from build123d import *

# Parameters (mm, degrees)
SKETCH_1_W           = 14
SKETCH_1_H           = 22
EXTRUDE_1_DEPTH      = 5
SKETCH_2_OUTSIDE_W   = 21.31
SKETCH_2_OUTSIDE_H   = 29.31
SKETCH_2_OUTSIDE_W_2 = 11
SKETCH_2_OUTSIDE_H_2 = 19
CUT_EXTRUDE_1_DEPTH  = 3.5
SKETCH_3_W           = 8
SKETCH_3_H           = 16
CUT_EXTRUDE_2_DEPTH  = 3
SKETCH_4_W           = 5.5
SKETCH_4_H           = 5
EXTRUDE_2_DEPTH      = 1.5
FILLET_1_R           = 2
FILLET_2_R           = 1
EXTRUDE_3_DEPTH      = 4
SKETCH_6_W           = 1
SKETCH_6_H           = 5
CUT_EXTRUDE_3_DEPTH  = 0.01
SKETCH_7_W           = 3
SKETCH_7_H           = 11
CUT_EXTRUDE_4_DEPTH  = 1
FILLET_3_R           = 0.5


with BuildPart() as part:
    # 草图1 → 凸台-拉伸1 (new body)
    with BuildSketch(Plane.XY):
        Rectangle(SKETCH_1_W, SKETCH_1_H)
    extrude(amount=EXTRUDE_1_DEPTH)

    # 草图2 outside → 切除-拉伸1 (cut)
    with BuildSketch(Plane.XY.offset(5)):
        Rectangle(SKETCH_2_OUTSIDE_W, SKETCH_2_OUTSIDE_H)
        Rectangle(SKETCH_2_OUTSIDE_W_2, SKETCH_2_OUTSIDE_H_2, mode=Mode.SUBTRACT)
    extrude(amount=-CUT_EXTRUDE_1_DEPTH, mode=Mode.SUBTRACT)

    # 草图3 → 切除-拉伸2 (cut)
    with BuildSketch(Plane(origin=(0, 0, 0), x_dir=(-1, 0, 0), z_dir=(0, 0, -1))):
        Rectangle(SKETCH_3_W, SKETCH_3_H)
    extrude(amount=-CUT_EXTRUDE_2_DEPTH, mode=Mode.SUBTRACT)

    # 草图4 → 凸台-拉伸2 (add)
    with BuildSketch(Plane(origin=(0, 0, 0), x_dir=(-1, 0, 0), z_dir=(0, 0, -1))):
        with Locations((0, -13.5)):
            Rectangle(SKETCH_4_W, SKETCH_4_H)
    extrude(amount=-EXTRUDE_2_DEPTH)

    # 圆角1
    fillet_1_edges = [part.edges().sort_by_distance(p)[0] for p in [
        (-7, 11, 0.75),
        (7, 11, 0.75),
        (7, -11, 0.75),
        (-7, -11, 0.75),
        (5.5, -9.5, 3.25),
        (-5.5, -9.5, 3.25),
        (-5.5, 9.5, 3.25),
        (5.5, 9.5, 3.25),
    ]]
    fillet(fillet_1_edges, radius=FILLET_1_R)

    # 圆角2
    fillet_2_edges = [part.edges().sort_by_distance(p)[0] for p in [
        (4, -8, 1.5),
        (4, 8, 1.5),
        (-4, 8, 1.5),
        (-4, -8, 1.5),
        (-2.75, -16, 0.75),
        (2.75, -16, 0.75),
    ]]
    fillet(fillet_2_edges, radius=FILLET_2_R)

    # 草图5 → 凸台-拉伸3 (add)
    with BuildSketch(Plane(origin=(0, 0, 0), x_dir=(-1, 0, 0), z_dir=(0, 0, -1))):
        Polygon((-2, -11), (-0.5, -11), (-0.5, -9.5), (0.5, -9.5), (0.5, -11), (2, -11), (2, -12), (0.5, -12), (0.5, -13.5), (-0.5, -13.5), (-0.5, -12), (-2, -12), align=None)
    extrude(amount=EXTRUDE_3_DEPTH)

    # 草图6 → 切除-拉伸3 (cut)
    with BuildSketch(Plane.XY.offset(5)):
        with BuildLine():
            Line((-1.25, 2.165063509), (-1.75, 3.031088913))
            ThreePointArc((-1.75, 3.031088913), (0, -3.5), (1.75, 3.031088913))
            Line((1.75, 3.031088913), (1.25, 2.165063509))
            ThreePointArc((1.25, 2.165063509), (0, -2.5), (-1.25, 2.165063509))
        make_face()
        with Locations((0, 3)):
            Rectangle(SKETCH_6_W, SKETCH_6_H)
    extrude(amount=-CUT_EXTRUDE_3_DEPTH, mode=Mode.SUBTRACT)

    # 草图7 → 切除-拉伸4 (cut)
    with BuildSketch(Plane(origin=(0, 0, 0), x_dir=(-1, 0, 0), z_dir=(0, 0, -1))):
        with Locations((-5.5, 0)):
            Rectangle(SKETCH_7_W, SKETCH_7_H)
    extrude(amount=-CUT_EXTRUDE_4_DEPTH, mode=Mode.SUBTRACT)

    # 圆角3
    fillet_3_edges = [part.edges().sort_by_distance(p)[0] for p in [
        (2, -11.5, -4),
        (0, -13.5, -4),
        (-2, -11.5, -4),
        (0, -9.5, -4),
        (5.5, -5.5, 0),
        (5.5, 5.5, 0),
    ]]
    fillet(fillet_3_edges, radius=FILLET_3_R)


solid = part.part
Work out the finished part from the listing and answer in its coordinate system (mm). A direction names the side the tool comes from. Round coordinates to 2 decimals unless told otherwise and drop trailing zeros. Write each loop counter-clockwise with the first axis right and the second up, starting at its lowest first coordinate (ties: lowest second). Pieces come first, ordered by that corner, then holes. Notation, with made-up numbers: (75.5, 70) - (114.5, 70) arc R22 ccw to (114.5, 96) - close; hole circle Ø8 at (-15.5, 34.25). An arc over 180 degrees is marked (long way). Answer in a Markdown table with one row per item. Add a question column.
1. Find the intervals of material crossed by line 1 along Y through (x, z) = (0, 2.5); line 2 along X through (y, z) = (-2.5, 1.25); line 3 along Z through (x, y) = (4.75, 4.5), in increasing order. Write a range as from..to.
2. For faces 1 (the flat face through (-4, -11, 1)), 2 (the flat face through (-0.5, -13, -2)), 3 (the cylindrical face through (4.93, 8.9, 3.23)), 4 (the cylindrical face through (3.715, 7.699, 1.521)), determine the directions among +Z, -Z, +X, -X, +Y, -Y from which every point of the face is accessible in a straight line to the end or side of a thin tool.
3. A cutting plane is placed at C-C, the plane y = -4. Determine the outline of the cut face in (x, z), and give its area (3 significant figures).
4. Given pin 1 (1 mm diameter, centred on y = 3.5, z = 2.5, fed in from -X); pin 2 (1.5 mm diameter, centred on x = 6, y = 0.5, fed in from -Z); pin 3 (0.8 mm diameter, centred on x = -1.5, z = -1, fed in from -Y), each flat-ended and moving along its own axis, determine where each tip first touches the part or whether it passes through.
5. A cutting plane is placed at A-A, the plane z = -1.25. Determine the outline of the cut face in (x, y), and give its area (3 significant figures).
Worked out:
| question | item | result |
|---|---|---|
| 1 | line 1 | -9.5..-8, 8..9.5 |
| 1 | line 2 | -7..-4, 4..7 |
| 1 | line 3 | 1..5 |
| 2 | face 1 | +Z, -Z, -X, -Y |
| 2 | face 2 | -Z, -X, -Y |
| 2 | face 3 | +Z, +X, +Y |
| 2 | face 4 | -Z |
| 3 | outline | (-7, 0) - (-4, 0) - (-4, 3) - (4, 3) - (4, 1) - (7, 1) - (7, 1.5) - (5.5, 1.5) - (5.5, 5) - (-5.5, 5) - (-5.5, 1.5) - (-7, 1.5) - close |
| 3 | area | 32.5 mm^2 |
| 4 | pin 1 | x = -5.5 |
| 4 | pin 2 | z = 1 |
| 4 | pin 3 | y = -12 |
| 5 | outline | (-2, -12) - (-0.5, -12) - (-0.5, -13.5) - (0.5, -13.5) - (0.5, -12) - (2, -12) - (2, -11) - (0.5, -11) - (0.5, -9.5) - (-0.5, -9.5) - (-0.5, -11) - (-2, -11) - close |
| 5 | area | 7.00 mm^2 |
